```python
from build123d import *

# Parameters (mm, degrees)
F1_DEPTH = 8
F3_W     = 8
F3_H     = 8
F3_R     = 2.4
F4_DEPTH = 1.7
F5_R     = 2.4
F6_DEPTH = 1.7


with BuildPart() as f1:
    # F0 (on Front) → F1 (new body)
    with BuildSketch(Plane.XZ):
        Polygon((-2.4, 9.6), (-4, 9.6), (-4, 0), (4, 0), (4, 9.6), (2.4, 9.6), (2.4, 11.3), (-2.4, 11.3), align=None)
    extrude(amount=F1_DEPTH)

    # F3 (on plane+point) → F4 (cut, through all)
    with BuildSketch(Plane.XY.offset(11.3)):
        with Locations((0, -4)):
            Rectangle(F3_W, F3_H)
        with Locations((0, -4)):
            Circle(F3_R, mode=Mode.SUBTRACT)
    extrude(amount=-F4_DEPTH, mode=Mode.SUBTRACT)

    # F5 (on Top) → F6 (cut)
    with BuildSketch(Plane.XY):
        with Locations((0, -4)):
            Circle(F5_R)
    extrude(amount=F6_DEPTH, mode=Mode.SUBTRACT)

    # F8: F1 across plane


with BuildPart() as f1_1:
    add(f1.part)
    add(f1.part.mirror(Plane.YZ.offset(4)))

    # F10: F1 across plane


with BuildPart() as f1_2:
    add(f1_1.part)
    add(f1_1.part.mirror(Plane.YZ.offset(12)))

    # F12: F1 across plane


with BuildPart() as f1_3:
    add(f1_2.part)
    add(f1_2.part.mirror(Plane.YZ.offset(28)))

    # F13: F1 across face


with BuildPart() as f1_4:
    add(f1_3.part)
    add(f1_3.part.mirror(Plane(origin=(60, -4, 4.8), x_dir=(0, 1, 0), z_dir=(1, 0, 0))))


solid = f1_4.part
```
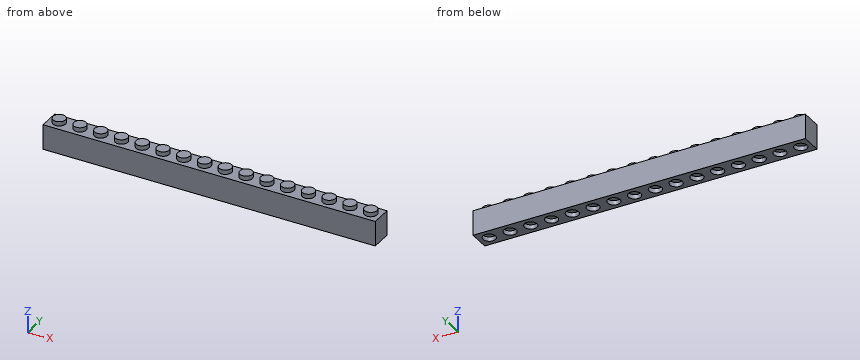
Geometry: final body of the model. Coordinates: model frame, mm. Round coordinates to 2 decimals unless told otherwise and drop trailing zeros. Order: outer loops, then holes, each group sorted by start corner. A loop starts at its lowest first (then second) coordinate and runs counter-clockwise, first axis right, second up. Notation, with made-up numbers: (51.5, 23) - (93.5, 23) arc R32 cw to (93.5, 50) - close; hole circle Ø10 at (81, 55). An arc over 180 degrees is marked (long way). Write item = value, one per line. Start each with the question number.
Q1. Ray query, line 1 (Z direction, x = 66, y = -0.5); line 2 (Y direction, x = 0, z = 0.95); line 3 (Z direction, x = 6, y = -5.25). Return the intervals inside material, ascending. Write a range as from..to.
Q2. Cut plane A-A on x = 120. Return the cut outline in (y, z).
Q3. Pin query (flat end, axial travel): pin 1 (3 mm diameter, centred on x = 73, y = -5, fed in from -Z); pin 2 (3 mm diameter, centred on x = 72, y = -4, fed in from -Z). Return the tip coordinate at first contact, or that it passes through.
Outcome:
q1.line_1 = 0..9.6
q1.line_2 = -8..-6.4, -1.6..0
q1.line_3 = 1.7..11.3
q2.outline = (-8, 0) - (-6.4, 0) - (-6.4, 1.7) - (-1.6, 1.7) - (-1.6, 0) - (0, 0) - (0, 9.6) - (-1.6, 9.6) - (-1.6, 11.3) - (-6.4, 11.3) - (-6.4, 9.6) - (-8, 9.6) - close
q3.pin_1 = 0
q3.pin_2 = 1.7
